Geometry check sheet. Reference: the model listing, model coordinates, mm. Face numbers are marked on the shaded views. Coordinates: 2 decimals unless noted, no trailing zeros. Order: outer loops, then holes, each group sorted by start corner. A loop starts at its lowest first (then second) coordinate and runs counter-clockwise, first axis right, second up. Notation, with made-up numbers: M -28.5,1 L 26.5,1 A25 ccw 26.5,20 Z; hole C 43,80 d11. An arc over 180 degrees is marked long. One line per item, written item: value. Start each with the question number.
1) Go/stop test with flat-tipped pins: P1, Ø3, axis at x = -5.5, y = 2, coming from the -Z side; P2, Ø3, axis at y = 3, z = -22.5, coming from the +X side; P3, Ø1.2, axis at x = 37.5, y = 4.5, coming from the -Z side; P4, Ø5, axis at x = 25.4, z = 7.62, coming from the -Y side. Record where each tip stops, or that it passes through.
2) Sectioned sample at A-A, the plane x = -4.5. Enter the section's corners in (y, z) (3 decimals), then the cut area to 3 significant figures.
3) Draft check along X on the marked faces 1, 2 and 3. Enter one of: pulls with the +X half, pulls with the -X half, needs draft (parallel to the pull), parting line crosses it, or undercut.
4) Sectioned sample at D-D, the plane z = -27. Enter the section's corners in (x, y).
5) Sectioned sample at B-B, the plane z = 5.5. Enter the section's corners in (x, y) (3 decimals), then the cut area to 3 significant figures.
6) Sectioned sample at C-C, the plane y = 4.5. State how many separate pieces and enclosed holes the cut face has, then the cut area to 3 significant figures.
7) Thickness scan on L1, parallel to X at y = 2.25, z = 7.62 (3 decimals); L2, parallel to Z at x = -7, y = 1.5; L3, parallel to Z at x = -27.5, y = 5.5. Record the ranges inside material, lowest first. Write a range as from..to.
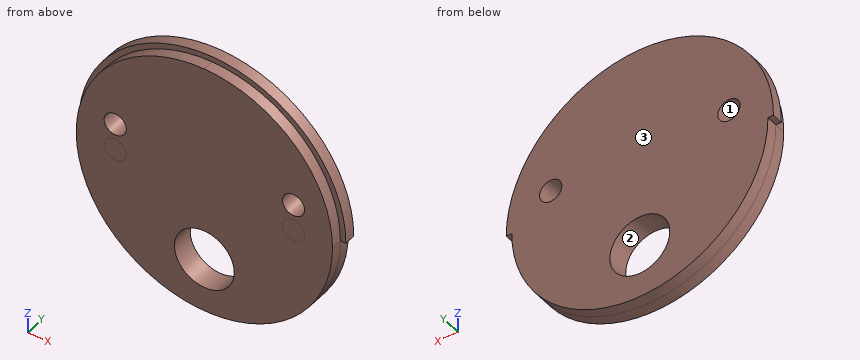
```python
from build123d import *

# Parameters (mm, degrees)
SKETCH1_R           = 36.5125
BOSS_EXTRUDE1_DEPTH = 3.175
SKETCH2_R           = 38.0746
BOSS_EXTRUDE2_DEPTH = 3.175
SKETCH3_R           = 5.08
CUT_EXTRUDE1_DEPTH  = 55.218749804
SKETCH7_R           = 3.175
CUT_EXTRUDE4_DEPTH  = 55.218749804
SKETCH8_R           = 8.5344
CUT_EXTRUDE5_DEPTH  = 55.218749804
BOSS_EXTRUDE3_START = -6.35
SKETCH9_R           = 3.175
BOSS_EXTRUDE3_DEPTH = 6.35
SKETCH10_R          = 3.175
CUT_EXTRUDE6_DEPTH  = 55.218749804


with BuildPart() as part:
    # Sketch1 → Boss-Extrude1 (new body)
    with BuildSketch(Plane(origin=(0, 0, 0), x_dir=(1, 0, 0), z_dir=(0, 1, 0))):
        with Locations(Location((0, 0, 0), (0, 0, 270))):
            Circle(SKETCH1_R)
    extrude(amount=BOSS_EXTRUDE1_DEPTH)

    # Sketch2 → Boss-Extrude2 (add)
    with BuildSketch(Plane(origin=(0, 3.175, 0), x_dir=(1, 0, 0), z_dir=(0, 1, 0))):
        with Locations(Location((0, 0, 0), (0, 0, 270))):
            Circle(SKETCH2_R)
    extrude(amount=BOSS_EXTRUDE2_DEPTH)

    # Sketch3 → Cut-Extrude1 (cut, through all)
    with BuildSketch(Plane.XZ):
        with Locations(Location((0, -20.9296, 0), (0, 0, 270))):
            Circle(SKETCH3_R)
    extrude(amount=-CUT_EXTRUDE1_DEPTH, mode=Mode.SUBTRACT)

    # Sketch7 → Cut-Extrude4 (cut, through all)
    with BuildSketch(Plane(origin=(0, 6.35, 0), x_dir=(1, 0, 0), z_dir=(0, 1, 0))):
        with Locations(Location((-25.4, 0, 0), (0, 0, 270))):
            Circle(SKETCH7_R)
        with Locations(Location((25.4, 0, 0), (0, 0, 270))):
            Circle(SKETCH7_R)
    extrude(amount=-CUT_EXTRUDE4_DEPTH, mode=Mode.SUBTRACT)

    # Sketch8 → Cut-Extrude5 (cut, through all)
    with BuildSketch(Plane.XZ):
        with Locations(Location((0, -20.9296, 0), (0, 0, 270))):
            Circle(SKETCH8_R)
        with BuildLine():
            Line((-38.0746, 0), (-36.5125, 0))
            ThreePointArc((-36.5125, 0), (0, -36.5125), (36.5125, 0))
            Line((36.5125, 0), (38.0746, 0))
            ThreePointArc((38.0746, 0), (0, -38.0746), (-38.0746, 0))
        make_face()
    extrude(amount=-CUT_EXTRUDE5_DEPTH, mode=Mode.SUBTRACT)

    # Sketch9 → Boss-Extrude3 (add)
    with BuildSketch(Plane.XZ.offset(BOSS_EXTRUDE3_START)):
        with Locations((-25.4, 0)):
            Circle(SKETCH9_R)
        with Locations((25.4, 0)):
            Circle(SKETCH9_R)
    extrude(amount=BOSS_EXTRUDE3_DEPTH)

    # Sketch10 → Cut-Extrude6 (cut, through all)
    with BuildSketch(Plane.XZ):
        with Locations(Location((-25.4, 7.62, 0), (0, 0, 270))):
            Circle(SKETCH10_R)
        with Locations(Location((25.4, 7.62, 0), (0, 0, 270))):
            Circle(SKETCH10_R)
    extrude(amount=-CUT_EXTRUDE6_DEPTH, mode=Mode.SUBTRACT)


solid = part.part
```
Final values:
1. P1: stops at z = -36.29
1. P2: stops at x = 29.87
1. P3: stops at z = 0
1. P4: passes through
2. outline: M 0,-36.234 L 6.35,-36.234 L 6.35,-28.181 L 0,-28.181 Z; M 0,-13.678 L 6.35,-13.678 L 6.35,37.808 L 3.175,37.808 L 3.175,36.234 L 0,36.234 Z
2. area: 373 mm^2
3. face 1: undercut
3. face 2: undercut
3. face 3: needs draft
4. outline: M -24.58,0 L -6,0 L -6,6.35 L -24.58,6.35 Z; M 6,0 L 24.58,0 L 24.58,6.35 L 6,6.35 Z
5. outline: M -37.675,3.175 L -36.096,3.175 L -36.096,0 L -27.764,0 L -27.764,6.35 L -37.675,6.35 Z; M -23.036,0 L 23.036,0 L 23.036,6.35 L -23.036,6.35 Z; M 27.764,0 L 36.096,0 L 36.096,3.175 L 37.675,3.175 L 37.675,6.35 L 27.764,6.35 Z
5. area: 408 mm^2
6. separate pieces: 1
6. enclosed holes: 3
6. area: 4,080 mm^2
7. L1: x = -35.709..-28.575, -22.225..22.225, 28.575..35.709
7. L2: z = -35.84..-25.81, -16.05..35.84
7. L3: z = -24.02..5.24, 10..26.33
